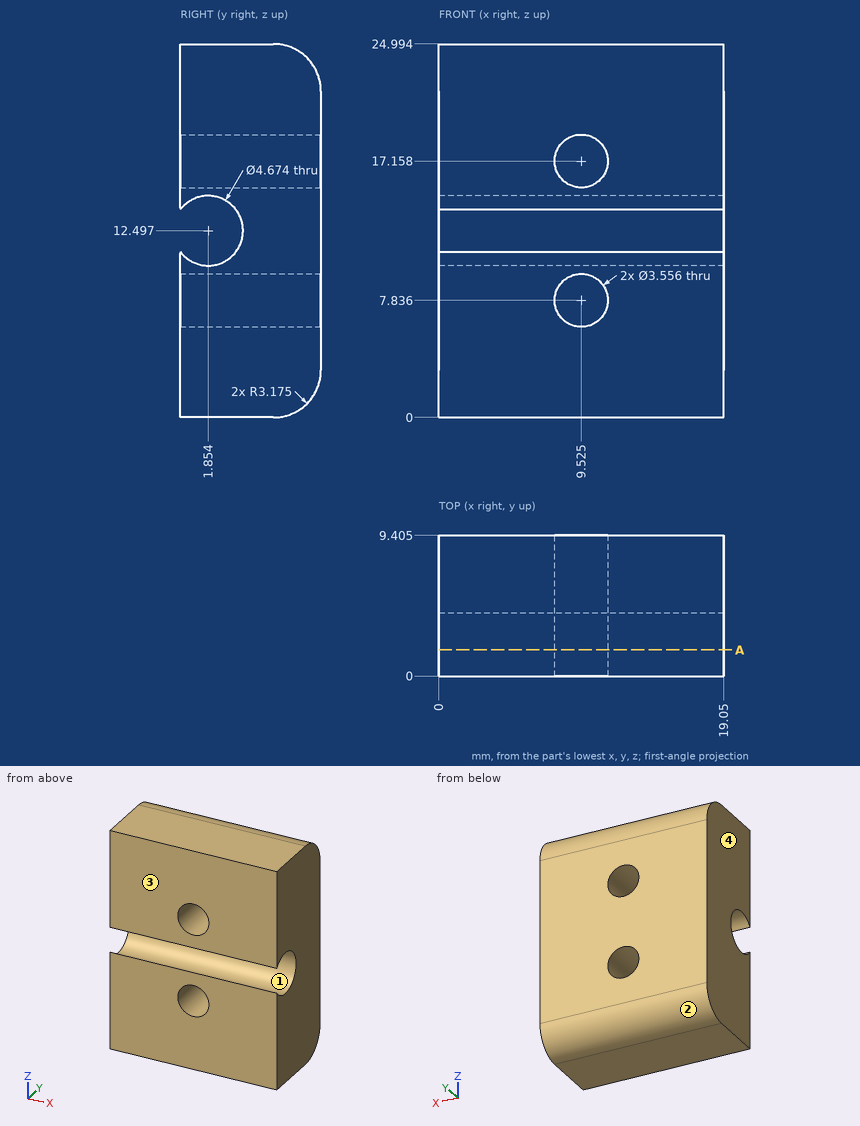
Input: dimensioned drawing with shaded views. Units: mm. Origin: part minimum x, y, z. Round coordinates to 2 decimals unless told otherwise and drop trailing zeros. Use CSV: the item, a comma, the result in double quotes. Start each with the question number.
Q1. Pull-direction query (Y, two-part tool) for the marked faces 1, 2, 3 and 4; classes: pulls with the +Y half, pulls with the -Y half, needs draft (parallel to the pull), parting line crosses it, or undercut.
Q2. Section A-A (y = 1.75). Give the number of separate pieces and of enclosed holes in the cut face, plus the area to 3 significant figures.
Q3. Line query: L1, parallel to Z at x = 12.5, y = 1.75; L2, parallel to X at y = 2.25, z = 17.25; L3, parallel to Z at x = 9.5, y = 8.5 (1 decimal). Output: solid intervals per line, ascending.
Result sheet:
1,face 1,"undercut"
1,face 2,"pulls with the +Y half"
1,face 3,"pulls with the -Y half"
1,face 4,"needs draft"
2,separate pieces,"2"
2,enclosed holes,"2"
2,area,"367 mm²"
3,L1,"0 to 10.16, 14.83 to 24.99"
3,L2,"0 to 7.75, 11.3 to 19.05"
3,L3,"1 to 6.1, 9.6 to 15.4, 18.9 to 24"
